from build123d import *

# Parameters (mm, degrees)
SKETCH1_R           = 1.5025
BOSS_EXTRUDE1_DEPTH = 3.25


with BuildPart() as part:
    # Sketch1 → Boss-Extrude1 (new body)
    with BuildSketch(Plane(origin=(0, 0, 0), x_dir=(1, 0, 0), z_dir=(0, 1, 0))):
        with BuildLine():
            Line((-14.5, 4), (14.5, 4))
            ThreePointArc((14.5, 4), (17.328427125, 2.828427125), (18.5, 0))
            Line((18.5, 0), (18.5, -4))
            Line((18.5, -4), (16.416864937, -4))
            ThreePointArc((16.416864937, -4), (15, -2.9975), (13.583135063, -4))
            Line((13.583135063, -4), (11.416864937, -4))
            ThreePointArc((11.416864937, -4), (10, -2.9975), (8.583135063, -4))
            Line((8.583135063, -4), (6.416864937, -4))
            ThreePointArc((6.416864937, -4), (5, -2.9975), (3.583135063, -4))
            Line((3.583135063, -4), (1.416864937, -4))
            ThreePointArc((1.416864937, -4), (0, -2.9975), (-1.416864937, -4))
            Line((-1.416864937, -4), (-3.583135063, -4))
            ThreePointArc((-3.583135063, -4), (-5, -2.9975), (-6.416864937, -4))
            Line((-6.416864937, -4), (-8.583135063, -4))
            ThreePointArc((-8.583135063, -4), (-10, -2.9975), (-11.416864937, -4))
            Line((-11.416864937, -4), (-13.583135063, -4))
            ThreePointArc((-13.583135063, -4), (-15, -2.9975), (-16.416864937, -4))
            Line((-16.416864937, -4), (-18.5, -4))
            Line((-18.5, -4), (-18.5, 0))
            ThreePointArc((-18.5, 0), (-17.328427125, 2.828427125), (-14.5, 4))
        make_face()
        with Locations((-15, 0.5)):
            Circle(SKETCH1_R, mode=Mode.SUBTRACT)
        with Locations((-10, 0.5)):
            Circle(SKETCH1_R, mode=Mode.SUBTRACT)
        with Locations((-5, 0.5)):
            Circle(SKETCH1_R, mode=Mode.SUBTRACT)
        with Locations((0, 0.5)):
            Circle(SKETCH1_R, mode=Mode.SUBTRACT)
        with Locations((5, 0.5)):
            Circle(SKETCH1_R, mode=Mode.SUBTRACT)
        with Locations((10, 0.5)):
            Circle(SKETCH1_R, mode=Mode.SUBTRACT)
        with Locations((15, 0.5)):
            Circle(SKETCH1_R, mode=Mode.SUBTRACT)
    extrude(amount=BOSS_EXTRUDE1_DEPTH)


solid = part.part
Can you work these out from the model? Positions are in its coordinate system, mm. Give positions to 0.01 mm unless a question says otherwise; leave off trailing zeros. Order: outer loops, then holes, each group sorted by start corner. A loop starts at its lowest first (then second) coordinate and runs counter-clockwise, first axis right, second up. Notation, with made-up numbers: (-2, 30.5) - (12, 30.5) arc R20 cw to (12, 53.5) - close; hole circle Ø6 at (70.25, 0). An arc over 180 degrees is marked (long way). Write each question's results on one line, items separated by ' | '.
1) If we mould it in two halves opening along Z, with no side actions, what happens to faces 1 (the face through (6.433, 1.602, -0.951)), 2 (the face through (8, 2, 4)), 3 (the face through (0, 2, -4)), 4 (the face through (18.5, 2, 2))? For each: pulls with the +Z half, pulls with the -Z half, needs draft (parallel to the pull), parting line crosses it, or undercut.
Final values:
face 1: undercut | face 2: pulls with the +Z half | face 3: pulls with the -Z half | face 4: needs draft
2) Suppose I cut it at B-B, the plane z = -1. Give the number of separate pieces and of enclosed holes in the cut face, then the cut area to 3 significant figures.
Final values:
separate pieces: 8 | enclosed holes: 0 | area: 55.0 mm^2
3) Please list where these lines run through material, in increasing order: line 1 along Z through (x, y) = (5, 1.6); line 2 along Z through (x, y) = (4, 3.05); line 3 along X through (y, z) = (0.35, -2.5). Write a range as [from, to].
Final values:
line 1: z = [-4, -2], [1, 3] | line 2: z = [-4, -1.62], [0.62, 3.38] | line 3: x = [-17.62, 17.62]
4) Suppose I cut it at C-C, the plane y = 0.4. Write out the boundary of the cut face in (x, z) (1 decimal), then the cut area to 3 significant figures.
Final values:
outline: (-18.5, 0) arc R4 ccw to (-14.5, -4) - (14.5, -4) arc R4 ccw to (18.5, 0) - (18.5, 4) - (16.4, 4) arc R1.5 cw to (13.6, 4) - (11.4, 4) arc R1.5 cw to (8.6, 4) - (6.4, 4) arc R1.5 cw to (3.6, 4) - (1.4, 4) arc R1.5 cw to (-1.4, 4) - (-3.6, 4) arc R1.5 cw to (-6.4, 4) - (-8.6, 4) arc R1.5 cw to (-11.4, 4) - (-13.6, 4) arc R1.5 cw to (-16.4, 4) - (-18.5, 4) - close; hole circle Ø3 at (-15, -0.5); hole circle Ø3 at (-10, -0.5); hole circle Ø3 at (-5, -0.5); hole circle Ø3 at (0, -0.5); hole circle Ø3 at (5, -0.5); hole circle Ø3 at (10, -0.5); hole circle Ø3 at (15, -0.5) | area: 225 mm^2
5) Suppose I cut it at D-D, the plane x = -15. Write out the boundary of the cut face in (y, z), then the cut area to 3 significant figures.
Final values:
outline: (0, -3.97) - (3.25, -3.97) - (3.25, -2) - (0, -2) - close; (0, 1) - (3.25, 1) - (3.25, 3) - (0, 3) - close | area: 12.9 mm^2
6) I'm going to push a flat-ended pin straight in: pin 1 Ø2.5 at (x, z) = (-15, -0.5) entering from +Y. Where does the tip first touch, or does it pass through?
Final values:
pin 1: passes through
7) Suppose I cut it at A-A, the plane x = 0. Write out the boundary of the cut face in (y, z).
Final values:
outline: (0, -4) - (3.25, -4) - (3.25, -2) - (0, -2) - close; (0, 1) - (3.25, 1) - (3.25, 3) - (0, 3) - close
